Source: CAD feature listing. Evaluate the final solid. Frame: model axes, mm. A direction names the side the tool comes from. Give positions to 0.01 mm unless a question says otherwise; leave off trailing zeros. Loops run counter-clockwise (first coordinate to the right, second up) from the corner with the lowest first, then second, coordinate; pieces in that order, holes last. Notation, with made-up numbers: (-2, -35.75) - (34, -35.75) arc R21 cw to (34, -14.75) - close; hole circle Ø4 at (-1.5, 66). An arc over 180 degrees is marked (long way). Write each question's results on one line, items separated by ' | '. Start each with the question number.
(1) Reachability of faces 1 (the flat face through (20, 1, -20)), 2 (the cylindrical face through (46.72, 0.99, 63.25)), 3 (the cylindrical face through (63.25, 0.99, -46.72)), 4 (the cylindrical face through (-63.25, 0.99, 46.72)), 5 (the cylindrical face through (-46.72, 0.99, -63.25)) from +Z, -Z, +X, -X, +Y, -Y: full face, straight path, thin tool, end or side. Return the list, or none.
(2) Material intervals for line 1 along X through (y, z) = (1.6, 5.5); line 2 along X through (y, z) = (0.95, -24.5), sorted ascending. Write a range as [from, to].
(3) Pull-direction query (Z, two-part tool) for faces 6 (the cylindrical face through (-107.6, 1, 106.9)), 7 (the cylindrical face through (47.598, 0.986, -64.164)), 8 (the flat face through (1, 2, -1)); classes: pulls with the +Z half, pulls with the -Z half, needs draft (parallel to the pull), parting line crosses it, or undercut.
(4) Contact query for flat-ended pins moving along their axis: pin 1 (3 mm diameter, centred on x = -52.59, z = -52.59, fed in from +Y); pin 2 (1 mm diameter, centred on y = 1, z = 7.5, fed in from +X); pin 3 (1 mm diameter, centred on x = 8.5, y = 1, fed in from +Z); pin 4 (1 mm diameter, centred on y = 0.5, z = -14, fed in from -X). Output: stop coordinate, or through.
(5) Cut plane C-C on y = 0.3. Give the number of separate pieces and of enclosed holes in the cut face, then the cut area to 3 significant figures.
(6) Cut plane B-B on z = -84.5. Return the cut outline in (x, y), then the cut area to 3 significant figures.
(7) Cut plane A-A on z = 68. Return the cut outline in (x, y), then the cut area to 3 significant figures.
from build123d import *

# Parameters (mm, degrees)
SKETCH2_R           = 4
SKETCH2_R_2         = 1
BOSS_EXTRUDE1_DEPTH = 2
CIRPATTERN1_COUNT   = 4


with BuildPart() as part:
    # Sketch2 → Boss-Extrude1 (new body)
    with BuildSketch(Plane(origin=(0, 0, 0), x_dir=(1, 0, 0), z_dir=(0, 1, 0))):
        with BuildLine():
            Line((0, 0), (35, 0))
            Line((35, 0), (35, 12.071067812))
            ThreePointArc((35, 12.071067812), (63.703714022, 47.158503121), (99.989485852, 74.331542663))
            ThreePointArc((99.989485852, 74.331542663), (107.253909229, 107.253909229), (74.331542663, 99.989485852))
            ThreePointArc((74.331542663, 99.989485852), (47.158503121, 63.703714022), (12.071067812, 35))
            Line((12.071067812, 35), (0, 35))
            Line((0, 35), (0, 0))
        make_face()
        with Locations((93.111773605, 93.111773605)):
            Circle(SKETCH2_R, mode=Mode.SUBTRACT)
        with Locations((52.588388778, 52.588388778)):
            Circle(SKETCH2_R_2, mode=Mode.SUBTRACT)
        with Locations((16.464466094, 30.606601718)):
            Circle(SKETCH2_R_2, mode=Mode.SUBTRACT)
        with Locations((30.606601718, 16.464466094)):
            Circle(SKETCH2_R_2, mode=Mode.SUBTRACT)
        with Locations((97.060009194, 77.261019321)):
            Circle(SKETCH2_R_2, mode=Mode.SUBTRACT)
        with Locations((77.261019321, 97.060009194)):
            Circle(SKETCH2_R_2, mode=Mode.SUBTRACT)
        with Locations((104.425482104, 104.425482104)):
            Circle(SKETCH2_R_2, mode=Mode.SUBTRACT)
        Polygon((5, 30), (5, 5), (30, 5), (30, 10), (10, 30), align=None, mode=Mode.SUBTRACT)
    boss_extrude1 = extrude(amount=BOSS_EXTRUDE1_DEPTH)

    # CirPattern1: Boss-Extrude1 ×4 about axis
    cirpattern1_axis = Axis((0, 0, 0), (0, 1, 0))
    for i in range(1, CIRPATTERN1_COUNT):
        add(boss_extrude1.rotate(cirpattern1_axis, i * 360 / CIRPATTERN1_COUNT))


solid = part.part
Ans:
1) face 1: +Y, -Y | face 2: +Z, +Y, -Y | face 3: +X, +Y, -Y | face 4: -X, +Y, -Y | face 5: -Z, +Y, -Y
2) line 1: [-35, -30], [-5, 5], [30, 35] | line 2: [-43.59, -15.5], [-5, 5], [15.5, 43.59]
3) face 6: undercut | face 7: pulls with the -Z half | face 8: needs draft
4) pin 1: y = 2 | pin 2: x = 35 | pin 3: z = 35 | pin 4: x = -36.56
5) separate pieces: 1 | enclosed holes: 32 | area: 15,400 mm^2
6) outline: (-111.16, 0) - (-64.39, 0) - (-64.39, 2) - (-111.16, 2) - close; (64.39, 0) - (111.16, 0) - (111.16, 2) - (64.39, 2) - close | area: 187 mm^2
7) outline: (-89.75, 0) - (-51.15, 0) - (-51.15, 2) - (-89.75, 2) - close; (51.15, 0) - (89.75, 0) - (89.75, 2) - (51.15, 2) - close | area: 154 mm^2
